Autodesk Inventor part; units mm, degrees
ref_plane "YZ Plane" through (0, 0, 0) normal (1, 0, 0) x (0, 1, 0)
ref_plane "XZ Plane" through (0, 0, 0) normal (0, 1, 0) x (-1, 0, 0)
ref_plane "XY Plane" through (0, 0, 0) normal (0, 0, 1) x (1, 0, 0)
sketch "Sketch1" plane through (0, 0, 0) normal (0, 0, 1) x (1, 0, 0)
  line L0 (0, 0) -> (-75, 0)
  line L1 (-75, 28) -> (0, 28)
  line L2 (0, 28) -> (0, 19.25) construction
  line L3 (0, 17) -> (-75, 17) construction
  line L4 (0, 17) -> (-4, 17) construction
  arc A0 (-4, 19.25) -> (-4, 14.75) centre (-4, 17) ccw
  line L5 (-4, 19.25) -> (0, 19.25)
  line L6 (-4, 14.75) -> (0, 14.75)
  line L7 (0, 28) -> (0, 19.25)
  line L8 (0, 14.75) -> (0, 0)
  line L9 (-37.5, 28) -> (-37.5, 0) construction
  arc A1 (-71, 14.75) -> (-71, 19.25) centre (-71, 17) ccw
  line L10 (-71, 19.25) -> (-75, 19.25)
  line L11 (-71, 14.75) -> (-75, 14.75)
  line L12 (-75, 0) -> (-75, 14.75)
  line L13 (-75, 19.25) -> (-75, 28)
  dimension "d0" = 75
  dimension "d1" = 28
  dimension "d2" = 11
  dimension "d3" = 4
  dimension "d4" = 4.5
extrude "Extrusion1" add sketch "Sketch1" along normal blind 3
fillet "Fillet1" radius 1 7 edges at (-37.5, 28, 3) (0, 28, 1.5) (-75, 28, 1.5) (0, 23.625, 3) (0, 7.375, 3) (-75, 23.625, 3) (-75, 7.375, 3)
properties part number "MirrorControllerModel" material "Iron, Cast"
Check sheet for the modelled part. Datum: model origin and axes. Units: mm. A direction names the side the tool comes from. Give positions to 0.01 mm unless a question says otherwise; leave off trailing zeros. Loops run counter-clockwise (first coordinate to the right, second up) from the corner with the lowest first, then second, coordinate; pieces in that order, holes last. Notation, with made-up numbers: M 22,-11 L 78,-11 A25 cw 78,2 Z; hole C 41.25,39 d2. An arc over 180 degrees is marked long. Return JSON: item names as keys, results as strings. Group by question number.
1. Cross-section at A-A on z = 1.45. Record the boundary of the cut face in (x, y), plus the area to 3 significant figures.
2. Thickness scan on L1, parallel to Y at x = -66, z = 2.1; L2, parallel to X at y = 8, z = 2.4; L3, parallel to X at y = 18.25, z = 0.25. Record the ranges inside material, lowest first.
3. Tool access check on faces 1 (the flat face through (-2, 14.75, 1)), 2 (the flat face through (0, 23, 1)), 3 (the flat face through (-73, 19.25, 1)). Record the directions out of +Z, -Z, +X, -X, +Y, -Y that give a thin tool (end or side, any length) a straight path to the whole face; none if there is none.
4. Cross-section at B-B on y = 17. Record the boundary of the cut face in (x, z), plus the area to 4 significant figures.
5. Mould release check, pull along Y, two halves, no side actions. Record for faces 4 (the flat face through (-73, 14.75, 1)), 5 (the flat face through (-2, 19.25, 1)), 6 (the flat face through (-38, 28, 1)), 7 (the flat face through (0, 7, 1)): released by +Y, released by -Y, zero draft, split by the parting line, or undercut.
Return value:
{
 "1": {"outline": "M -75,0 L 0,0 L 0,14.75 L -4,14.75 A2.25 cw -4,19.25 L 0,19.25 L 0,27 A1 ccw -1,28 L -74,28 A1 ccw -75,27 L -75,19.25 L -71,19.25 A2.25 cw -71,14.75 L -75,14.75 Z", "area": "2,050 mm^2"},
 "2": {"L1": "0 to 27.99", "L2": "-74.92 to -0.08", "L3": "-69.13 to -5.87"},
 "3": {"face 1": "+Z, -Z, +X", "face 2": "+Z, -Z, +X, +Y, -Y", "face 3": "+Z, -Z, -X"},
 "4": {"outline": "M -68.75,0 L -6.25,0 L -6.25,3 L -68.75,3 Z", "area": "187.5 mm^2"},
 "5": {"face 4": "undercut", "face 5": "undercut", "face 6": "released by +Y", "face 7": "zero draft"}
}
